from build123d import *

# Parameters (mm, degrees)
F0_R     = 9.5
F0_R_2   = 5.25
F1_DEPTH = 10
F2_R     = 5.25
F2_R_2   = 3
F3_DEPTH = 5
F5_DEPTH = 12.5


with BuildPart() as f1:
    # F0 (on Top) → F1 (new body)
    with BuildSketch(Plane.XY):
        Circle(F0_R)
        Circle(F0_R_2, mode=Mode.SUBTRACT)
    extrude(amount=F1_DEPTH)

    # F2 (on Top) → F3 (join)
    with BuildSketch(Plane.XY):
        Circle(F2_R)
        Circle(F2_R_2, mode=Mode.SUBTRACT)
    extrude(amount=F3_DEPTH)

    # F4 (on Front) → F5 (intersect, symmetric)
    with BuildSketch(Plane.XZ):
        Polygon((25, 8), (-25, 10), (-25, 0), (25, 0), align=None)
    extrude(amount=F5_DEPTH, both=True, mode=Mode.INTERSECT)


solid = f1.part
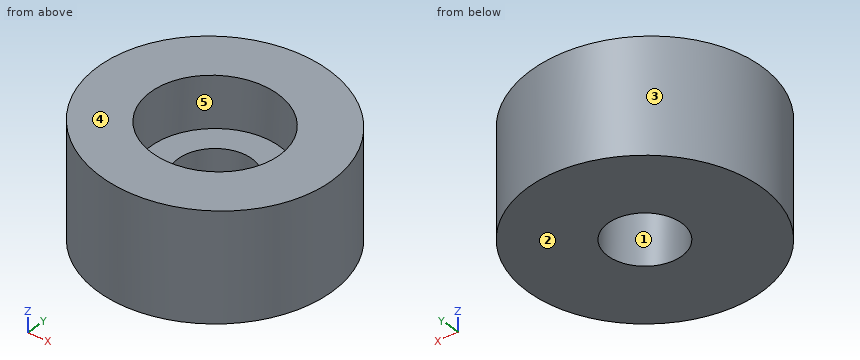
Here's how the part is built. I have some questions about the finished solid (model axes, mm). Face numbers are marked on the shaded views. A direction names the side the tool comes from. Give positions to 0.01 mm unless a question says otherwise; leave off trailing zeros. Order: outer loops, then holes, each group sorted by start corner. A loop starts at its lowest first (then second) coordinate and runs counter-clockwise, first axis right, second up. Notation, with made-up numbers: M 75,-36.5 L 109,-36.5 A29 cw 109,-16.5 Z; hole C 62,35.25 d9. An arc over 180 degrees is marked long. Answer as a JSON object with one key per item and string values. Group by question number.
1) Suppose I cut it at A-A, the plane x = 0. Write out the boundary of the cut face in (y, z).
2) Suppose I cut it at C-C, the plane z = 8.25. Write out the boundary of the cut face in (x, y).
3) Suppose I cut it at B-B, the plane y = 0. Write out the boundary of the cut face in (x, z).
4) I'm going to push flat-ended pins straight in: pin 1 Ø6 at (x, y) = (-1.5, -2) entering from +Z; pin 2 Ø6.5 at (x, y) = (0, 0) entering from -Z; pin 3 Ø2 at (x, z) = (-3, 3) entering from +Y. Where does each tip first touch, or does it pass through?
5) Please list where these lines run through material, in increasing order: L1, parallel to X at y = 0, z = 7.6; L2, parallel to Y at x = 0, z = 2.5. Write a range as [from, to].
6) Suppose I cut it at D-D, the plane y = 4.25. Write out the boundary of the cut face in (x, z).
7) On a 3-axis mill with a long thin cutter (end or side, diameter ignored), from which of +Z, -Z, +X, -X, +Y, -Y can I reach the whole of each face in a straight line? I mean the marked faces 4 and 5. Say none if no direction works.
8) We'd pull the mould along X, two halves only. Please class the marked faces 1, 2 and 3: pulls with the +X half, pulls with the -X half, needs draft (parallel to the pull), parting line crosses it, or undercut.
Results found:
{
 "1": {"outline": "M -9.5,0 L -3,0 L -3,5 L -5.25,5 L -5.25,9 L -9.5,9 Z; M 3,0 L 9.5,0 L 9.5,9 L 5.25,9 L 5.25,5 L 3,5 Z"},
 "2": {"outline": "C 0,0 d19; hole C 0,0 d10.5"},
 "3": {"outline": "M -9.5,0 L -3,0 L -3,5 L -5.25,5 L -5.25,9.21 L -9.5,9.38 Z; M 3,0 L 9.5,0 L 9.5,8.62 L 5.25,8.79 L 5.25,5 L 3,5 Z"},
 "4": {"pin 1": "z = 9.17", "pin 2": "z = 0", "pin 3": "y = 9.29"},
 "5": {"L1": "[-9.5, -5.25], [5.25, 9.5]", "L2": "[-9.5, -3], [3, 9.5]"},
 "6": {"outline": "M -8.5,0 L 8.5,0 L 8.5,8.66 L 3.08,8.88 L 3.08,5 L -3.08,5 L -3.08,9.12 L -8.5,9.34 Z"},
 "7": {"face 4": "+Z, +X, +Y, -Y", "face 5": "+Z"},
 "8": {"face 1": "undercut", "face 2": "needs draft", "face 3": "parting line crosses it"}
}
